```python
from build123d import *

# Parameters (mm, degrees)
SKETCH1_R           = 32.5
BOSS_EXTRUDE1_DEPTH = 300
SKETCH2_W           = 14
SKETCH2_H           = 44
CUT_EXTRUDE1_DEPTH  = 10


with BuildPart() as part:
    # Sketch1 → Boss-Extrude1 (new body)
    with BuildSketch(Plane(origin=(0, 0, 0), x_dir=(1, 0, 0), z_dir=(0, 1, 0))):
        with Locations(Location((0, 0, 0), (0, 0, 270))):
            Circle(SKETCH1_R)
    extrude(amount=BOSS_EXTRUDE1_DEPTH)

    # Sketch2 → Cut-Extrude1 (cut)
    with BuildSketch(Plane.ZY.offset(32.5)):
        with Locations((0, 251.6)):
            Rectangle(SKETCH2_W, SKETCH2_H)
    extrude(amount=-CUT_EXTRUDE1_DEPTH, mode=Mode.SUBTRACT)


solid = part.part
```
Can you work these out from the model? Positions are in its coordinate system, mm. A direction names the side the tool comes from. Coordinates: 2 decimals unless noted, no trailing zeros. Loops run counter-clockwise (first coordinate to the right, second up) from the corner with the lowest first, then second, coordinate; pieces in that order, holes last. Notation, with made-up numbers: M 56.5,-30.75 L 100.5,-30.75 A23 cw 100.5,-1.75 Z; hole C -25,31.25 d9. An arc over 180 degrees is marked long. Put each result on its own line as item: value. Start each with the question number.
(1) We'd pull the mould along Z, two halves only. Please class faces 1 (the face through (0, 0, 0)), 2 (the face through (-28, 273.6, 0)), 3 (the face through (9.76, 147.9, 31)): +Z half, -Z half, draft (parallel to the pull), parting line (faces both ways), or undercut.
(2) I need wall thicknesses on probe 1 along Z at (x, y) = (-1, 283.5); probe 2 along Z at (x, y) = (25.5, 286.5); probe 3 along X at (y, z) = (134.5, 19). Which ranges of each line are inside material? Lowest first, please.
(3) Imagine slicing it at A-A on x = -28. List the corners of the cut face in (y, z) for me, and give its area (3 significant figures).
(4) Imagine slicing it at D-D on x = -17. List the corners of the cut face in (y, z) for me, and give its area (3 significant figures).
(5) Will these pins go through, and if not, where does the flat tip stop? pin 1 Ø4 at (y, z) = (252.5, 1) entering from -X; pin 2 Ø2 at (x, y) = (11.5, 225.5) entering from +Z; pin 3 Ø8 at (y, z) = (68.5, -5.5) entering from +X; pin 4 Ø5 at (x, z) = (-25.5, 14.5) entering from -Y.
(6) Which directions (+Z, -Z, +X, -X, +Y, -Y) give clear straight access to the entire face, cutting with the end or side of a thin tool? Please do faces 4 (the face through (-27, 251, -7)), 5 (the face through (0, 300, 0)).
(7) Imagine slicing it at B-B on z = 0. List the corners of the cut face in (x, y) for me, and give its area (3 significant figures).
(8) Imagine slicing it at C-C on y = 51. List the corners of the cut face in (x, z) for me, and give its area (3 significant figures).
Worked answers:
1. face 1: draft
1. face 2: undercut
1. face 3: parting line
2. probe 1: z = -32.48 to 32.48
2. probe 2: z = -20.15 to 20.15
2. probe 3: x = -26.37 to 26.37
3. outline: M 0,-16.5 L 300,-16.5 L 300,16.5 L 0,16.5 Z; hole M 229.6,-7 L 273.6,-7 L 273.6,7 L 229.6,7 Z
3. area: 9,280 mm2
4. outline: M 0,-27.7 L 300,-27.7 L 300,27.7 L 0,27.7 Z
4. area: 16,600 mm2
5. pin 1: stops at x = -22.5
5. pin 2: stops at z = 30.76
5. pin 3: stops at x = 32.47
5. pin 4: stops at y = 0
6. face 4: -X
6. face 5: +Z, -Z, +X, -X, +Y
7. outline: M -32.5,0 L 32.5,0 L 32.5,300 L -32.5,300 L -32.5,273.6 L -22.5,273.6 L -22.5,229.6 L -32.5,229.6 Z
7. area: 19,100 mm2
8. outline: C 0,0 d65
8. area: 3,320 mm2
